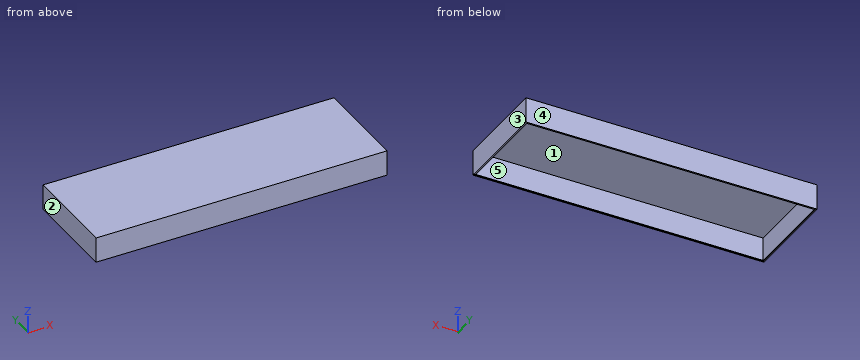
```python
from build123d import *

# Parameters (mm, degrees)
F0_W     = 304.8
F0_H     = 101.6
F0_W_2   = 301.6
F0_H_2   = 98.4
F1_DEPTH = 25
F2_W     = 304.8
F2_H     = 101.6
F3_DEPTH = 1.6
F4_W     = 0.644748
F4_H     = 0.498444
F5_DEPTH = 303.2
F6_W     = 0.51682
F6_H     = 0.5
F7_DEPTH = 100.644748


with BuildPart() as f1:
    # F0 (on Top) → F1 (new body)
    with BuildSketch(Plane.XY):
        with Locations((4.001044, -97.389185)):
            Rectangle(F0_W, F0_H)
        with Locations((4.001044, -97.389185)):
            Rectangle(F0_W_2, F0_H_2, mode=Mode.SUBTRACT)
    extrude(amount=F1_DEPTH)

    # F2 (on face) → F3 (join)
    with BuildSketch(Plane.XY.offset(25)):
        with Locations((4.001044, -97.389185)):
            Rectangle(F2_W, F2_H)
    extrude(amount=F3_DEPTH)

    # F4 (on face) → F5 (cut, through all)
    with BuildSketch(Plane.YZ.offset(-146.798956)):
        with Locations((-146.911559, 0.249222)):
            Rectangle(F4_W, F4_H)
    extrude(amount=F5_DEPTH, mode=Mode.SUBTRACT)

    # F6 (on face) → F7 (cut, through all)
    with BuildSketch(Plane(origin=(0, -147.233933, 0), x_dir=(-1, 0, 0), z_dir=(0, 1, 0))):
        with Locations((147.057366, 0.25)):
            Rectangle(F6_W, F6_H)
    extrude(amount=F7_DEPTH, mode=Mode.SUBTRACT)


solid = f1.part
```
CAD build for the part. Positions are in the model's coordinates, mm. Face numbers are marked on the shaded views. A direction names the side the tool comes from. Give positions to 0.01 mm unless a question says otherwise; leave off trailing zeros. Order: outer loops, then holes, each group sorted by start corner. A loop starts at its lowest first (then second) coordinate and runs counter-clockwise, first axis right, second up.
(1) Flat gauge pin, fed straight in: pin 1 (2 mm diameter, centred on x = -36, y = -110, fed in from -Z). Where does the tip first touch, or does it go through?
(2) Saw through at A-A, the plane z = 14.5. Give the cut face in (x, y).
(3) Drill centre lines: L1, parallel to X at y = -98.5, z = 22.5; L2, parallel to Y at x = 28, z = 21; L3, parallel to Z at x = 72, y = -131.5. Where is each one in solid material? Low to high.
(4) Mould opens along X. For the marked faces 1, 2 and 3 say: released by +X, released by -X, zero draft, split by the parting line, or undercut.
(5) Saw through at C-C, the plane y = -123.5. Give the cut face in (x, z), then the cut area to 3 significant figures.
(6) Saw through at B-B, the plane x = 7. Give the cut face in (y, z).
(7) Tool access for the marked faces 4 and 5: list every direction of +Z, -Z, +X, -X, +Y, -Y with a clear straight run to the whole face (end or side of a thin tool).
Results found:
1. pin 1: stops at z = 25
2. outline: (-148.4, -148.19) - (156.4, -148.19) - (156.4, -46.59) - (-148.4, -46.59) - close; hole (-146.8, -146.59) - (154.8, -146.59) - (154.8, -48.19) - (-146.8, -48.19) - close
3. L1: x = -148.4 to -146.8, 154.8 to 156.4
3. L2: y = -148.19 to -146.59, -48.19 to -46.59
3. L3: z = 25 to 26.6
4. face 1: undercut
4. face 2: released by -X
4. face 3: released by +X
5. outline: (-148.4, 0) - (-147.32, 0) - (-147.32, 0.5) - (-146.8, 0.5) - (-146.8, 25) - (154.8, 25) - (154.8, 0) - (156.4, 0) - (156.4, 26.6) - (-148.4, 26.6) - close
5. area: 567 mm2
6. outline: (-148.19, 0) - (-147.23, 0) - (-147.23, 0.5) - (-146.59, 0.5) - (-146.59, 25) - (-48.19, 25) - (-48.19, 0) - (-46.59, 0) - (-46.59, 26.6) - (-148.19, 26.6) - close
7. face 4: +Z, -Z, +X, -X, +Y
7. face 5: -Z
